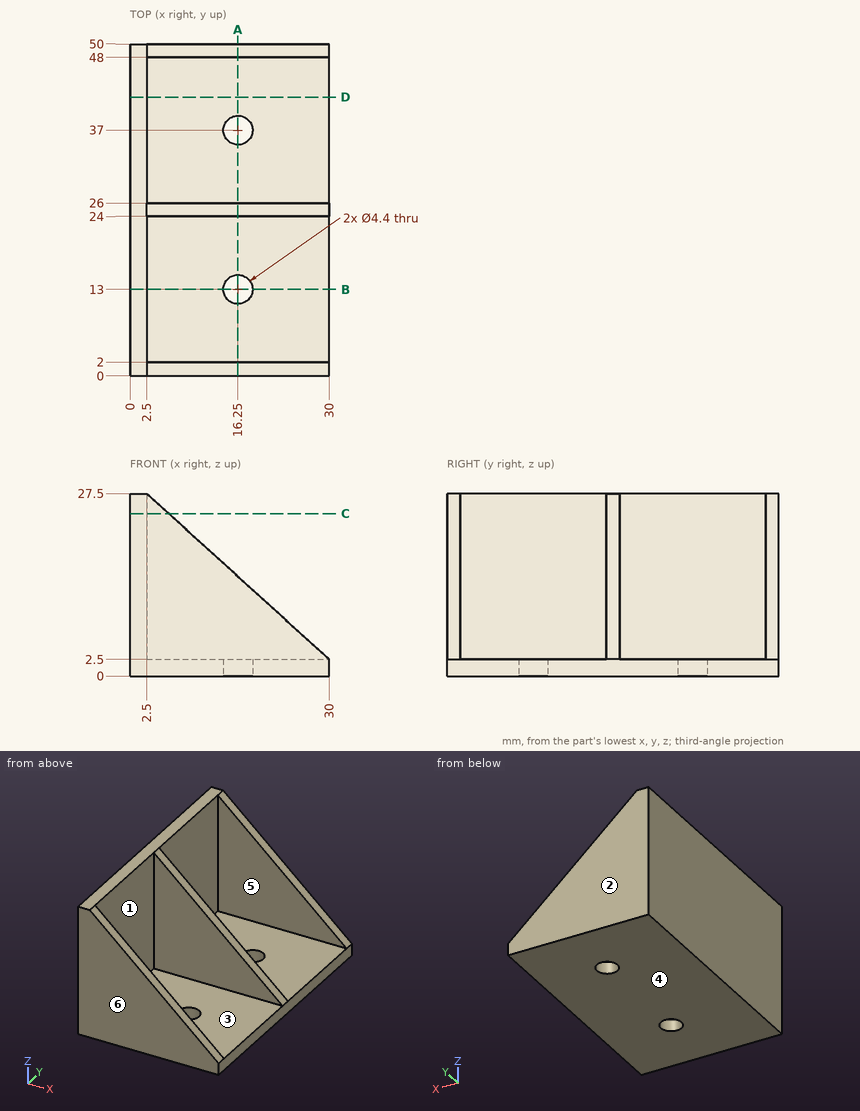
Answer from the drawing. Dimensions are ordinates in mm from the lowest x, y and z of the part. A direction names the side the tool comes from. Coordinates: 2 decimals unless noted, no trailing zeros. Order: outer loops, then holes, each group sorted by start corner. A loop starts at its lowest first (then second) coordinate and runs counter-clockwise, first axis right, second up. Notation, with made-up numbers: (-3, -5) -> (3, -5) arc R23 ccw to (3, 24) -> close; hole circle Ø9 at (-38.75, 5.25). An arc over 180 degrees is marked (long way). Answer as a JSON object with one key per item and string values.
1) A cutting plane is placed at B-B, the plane y = 13. Determine the outline of the cut face in (x, z), plus the area to 4 significant figures.
Model answer:
{"outline": "(0, 0) -> (14.05, 0) -> (14.05, 2.5) -> (2.5, 2.5) -> (2.5, 27.5) -> (0, 27.5) -> close; (18.45, 0) -> (30, 0) -> (30, 2.5) -> (18.45, 2.5) -> close", "area": "126.5 mm²"}
2) A cutting plane is placed at C-C, the plane z = 24.5. Determine the outline of the cut face in (x, y), plus the area to 3 significant figures.
Model answer:
{"outline": "(0, 0) -> (5.8, 0) -> (5.8, 2) -> (2.5, 2) -> (2.5, 24) -> (5.8, 24) -> (5.8, 26) -> (2.5, 26) -> (2.5, 48) -> (5.8, 48) -> (5.8, 50) -> (0, 50) -> close", "area": "145 mm²"}
3) A cutting plane is placed at A-A, the plane x = 16.25. Determine the outline of the cut face in (y, z), plus the area to 3 significant figures.
Model answer:
{"outline": "(0, 0) -> (10.8, 0) -> (10.8, 2.5) -> (2, 2.5) -> (2, 15) -> (0, 15) -> close; (15.2, 0) -> (34.8, 0) -> (34.8, 2.5) -> (26, 2.5) -> (26, 15) -> (24, 15) -> (24, 2.5) -> (15.2, 2.5) -> close; (39.2, 0) -> (50, 0) -> (50, 15) -> (48, 15) -> (48, 2.5) -> (39.2, 2.5) -> close", "area": "178 mm²"}
4) A tool of negligible diameter and unlimited length cuts with its end or side. For the marked faces 5 and 6, from which of +Z, -Z, +X, -X, +Y, -Y can it reach the whole face along a straight path? Write none if from no direction.
Model answer:
{"face 5": "+Z, +X", "face 6": "+Z, -Z, +X, -X, -Y"}
5) Consider line 1 along Y through (x, z) = (16.25, 1.1); line 2 along Y through (x, z) = (25, 6); line 3 along X through (y, z) = (37.5, 16). Determine where each line is inside the solid, lowest interval first. Write a range as from..to.
Model answer:
{"line 1": "y = 0..10.8, 15.2..34.8, 39.2..50", "line 2": "y = 0..2, 24..26, 48..50", "line 3": "x = 0..2.5"}
6) A cutting plane is placed at D-D, the plane y = 42. Determine the outline of the cut face in (x, z), plus the area to 4 significant figures.
Model answer:
{"outline": "(0, 0) -> (30, 0) -> (30, 2.5) -> (2.5, 2.5) -> (2.5, 27.5) -> (0, 27.5) -> close", "area": "137.5 mm²"}
7) Each of these flat-tipped pins is pushed along its axis until it touches: pin 1 (6.5 mm diameter, centred on y = 35.5, z = 21, fed in from +X); pin 2 (8 mm diameter, centred on x = 15.5, y = 13, fed in from +Z). Where does it stop, or does it pass through?
Model answer:
{"pin 1": "stops at x = 2.5", "pin 2": "stops at z = 2.5"}
8) The mould has two halves that part along Y. Classify the marked faces 1, 2, 3 and 4: released by +Y, released by -Y, zero draft, split by the parting line, or undercut.
Model answer:
{"face 1": "undercut", "face 2": "released by +Y", "face 3": "undercut", "face 4": "zero draft"}
